from build123d import *

# Parameters (mm, degrees)
EXTRUDE_1_DEPTH      = 13.5
SKETCH_5_R           = 10.1
CUT_EXTRUDE_2_DEPTH  = 1.5
SKETCH_7_R           = 3.5
CUT_EXTRUDE_3_DEPTH  = 37
SKETCH_9_R           = 1.5
CUT_EXTRUDE_4_DEPTH  = 24.5
SKETCH_11_W          = 60.4
SKETCH_11_H          = 24
EXTRUDE_2_DEPTH      = 10
SKETCH_12_R          = 2.7
CUT_EXTRUDE_5_DEPTH  = 8.5
SKETCH_18_R          = 12
CUT_EXTRUDE_9_DEPTH  = 1.5
SKETCH_19_W          = 14.67242397
SKETCH_19_H          = 6
CUT_EXTRUDE_10_DEPTH = 3
SKETCH_20_W          = 76.507524202
SKETCH_20_H          = 37.102074034
CUT_EXTRUDE_11_DEPTH = 3.5


with BuildPart() as part:
    # Sketch 1 → Extrude 1 (new body)
    with BuildSketch(Plane.XY):
        with BuildLine():
            Line((0, 12), (36.185307738, 12))
            Line((36.185307738, 12), (36.185307738, -12))
            Line((36.185307738, -12), (0, -12))
            ThreePointArc((0, -12), (-12, 0), (0, 12))
        make_face()
    extrude(amount=EXTRUDE_1_DEPTH)

    # Sketch 5 → Cut-Extrude 2 (cut)
    with BuildSketch(Plane(origin=(0, 0, 0), x_dir=(-1, 0, 0), z_dir=(0, 0, -1))):
        Circle(SKETCH_5_R)
    extrude(amount=-CUT_EXTRUDE_2_DEPTH, mode=Mode.SUBTRACT)

    # Sketch 7 → Cut-Extrude 3 (cut)
    with BuildSketch(Plane(origin=(0, 0, 1.5), x_dir=(-1, 0, 0), z_dir=(0, 0, -1))):
        Circle(SKETCH_7_R)
    extrude(amount=-CUT_EXTRUDE_3_DEPTH, mode=Mode.SUBTRACT)

    # Sketch 9 → Cut-Extrude 4 (cut)
    with BuildSketch(Plane(origin=(0, 0, 1.5), x_dir=(-1, 0, 0), z_dir=(0, 0, -1))):
        with Locations((-4.949747468, 4.949747468)):
            Circle(SKETCH_9_R)
        with Locations((4.949747468, 4.949747468)):
            Circle(SKETCH_9_R)
        with Locations((4.949747468, -4.949747468)):
            Circle(SKETCH_9_R)
        with Locations((-4.949747468, -4.949747468)):
            Circle(SKETCH_9_R)
    extrude(amount=-CUT_EXTRUDE_4_DEPTH, mode=Mode.SUBTRACT)


with BuildPart() as body_2:
    # Mirror 14: mirrored copy
    add(part.part.mirror(Plane(origin=(0, 0, -16.7), x_dir=(1, 0, 0), z_dir=(0, 0, -1))))


with BuildPart() as part_1:
    add(part.part)

    add(body_2.part)  # Extrude 2 merges body 2
    # Sketch 11 → Extrude 2 (add)
    with BuildSketch(Plane(origin=(36.185307738, 0, 0), x_dir=(0, 0, -1), z_dir=(1, 0, 0))):
        with Locations((16.7, 0)):
            Rectangle(SKETCH_11_W, SKETCH_11_H)
    extrude(amount=-EXTRUDE_2_DEPTH)

    # Sketch 12 → Cut-Extrude 5 (cut)
    with BuildSketch(Plane.XY.offset(13.5)):
        with Locations((4.949747468, 4.949747468)):
            Circle(SKETCH_12_R)
        with Locations((4.949747468, -4.949747468)):
            Circle(SKETCH_12_R)
        with Locations((-4.949747468, -4.949747468)):
            Circle(SKETCH_12_R)
        with Locations((-4.949747468, 4.949747468)):
            Circle(SKETCH_12_R)
    cut_extrude_5 = extrude(amount=-CUT_EXTRUDE_5_DEPTH, mode=Mode.SUBTRACT)

    # Sketch 18 → Cut-Extrude 9 (cut)
    with BuildSketch(Plane(origin=(0, 0, 0), x_dir=(-1, 0, 0), z_dir=(0, 0, -1))):
        Circle(SKETCH_18_R)
    cut_extrude_9 = extrude(amount=-CUT_EXTRUDE_9_DEPTH, mode=Mode.SUBTRACT)

    # Sketch 19 → Cut-Extrude 10 (cut)
    with BuildSketch(Plane(origin=(0, 0, 1.5), x_dir=(-1, 0, 0), z_dir=(0, 0, -1))):
        with Locations((7.336211985, 0)):
            Rectangle(SKETCH_19_W, SKETCH_19_H)
    cut_extrude_10 = extrude(amount=-CUT_EXTRUDE_10_DEPTH, mode=Mode.SUBTRACT)

    # Sketch 20 → Cut-Extrude 11 (cut)
    with BuildSketch(Plane.XY.offset(13.5)):
        with Locations((20.283666709, 0.248055891)):
            Rectangle(SKETCH_20_W, SKETCH_20_H)
    cut_extrude_11 = extrude(amount=-CUT_EXTRUDE_11_DEPTH, mode=Mode.SUBTRACT)

    # Mirror 24: Cut-Extrude 5, Cut-Extrude 9, Cut-Extrude 10 across plane
    add(cut_extrude_5.mirror(Plane(origin=(0, 0, -16.7), x_dir=(1, 0, 0), z_dir=(0, 0, -1))), mode=Mode.SUBTRACT)
    add(cut_extrude_9.mirror(Plane(origin=(0, 0, -16.7), x_dir=(1, 0, 0), z_dir=(0, 0, -1))), mode=Mode.SUBTRACT)
    add(cut_extrude_10.mirror(Plane(origin=(0, 0, -16.7), x_dir=(1, 0, 0), z_dir=(0, 0, -1))), mode=Mode.SUBTRACT)

    # Mirror 26: Cut-Extrude 11 across plane
    add(cut_extrude_11.mirror(Plane(origin=(0, 0, -16.7), x_dir=(1, 0, 0), z_dir=(0, 0, -1))), mode=Mode.SUBTRACT)


solid = part_1.part
Source: CAD feature listing. Evaluate the final solid. Frame: model axes, mm. A direction names the side the tool comes from. Give positions to 0.01 mm unless a question says otherwise; leave off trailing zeros. Write each loop counter-clockwise with the first axis right and the second up, starting at its lowest first coordinate (ties: lowest second). Pieces come first, ordered by that corner, then holes. Notation, with made-up numbers: (62, 40) - (95, 40) arc R6 cw to (95, 48) - close; hole circle Ø7 at (80, -35). An arc over 180 degrees is marked (long way). Write item = value, one per line. Start each with the question number.
Q1. Cut plane B-B, the plane x = 13.5. Return loops of the section in (y, z).
Q2. Cut plane C-C, the plane z = -37. Return loops of the section in (x, y).
Q3. Reachability of faces 4 (the cylindrical face through (6.14, 4.04, -36.63)), 5 (the flat face through (-8, 0, -37.9)), 6 (the cylindrical face through (4.364, -7.586, 7.535)), 7 (the flat face through (5, -7, -38.4)), 8 (the flat face through (19, 0, 0)) from +Z, -Z, +X, -X, +Y, -Y: full face, straight path, thin tool, end or side. Return the list, or none.
Q4. Pin query (flat end, axial travel): pin 1 Ø2.5 at (x, y) = (-5.5, -6) entering from +Z; pin 2 Ø2.5 at (x, z) = (-5.5, -37) entering from +Y; pin 3 Ø3.5 at (x, y) = (-4.95, 4.95) entering from -Z. Return the tip coordinate at first contact, or that it passes through.
Q5. Cut plane A-A, the plane y = 0. Return loops of the section in (x, z).
Q6. Material intervals for probe 1 along Z at (x, y) = (7, -0.5); probe 2 along Z at (x, y) = (24, 9.5); probe 3 along X at (y, z) = (-2.75, 7.5), sorted ascending.
Q7. Draft query along Y for faces 1 (the flat face through (-5, 3, -38.4)), 2 (the flat face through (17, 0, -43.4)), 3 (the flat face through (26.4, -12, -17.1)). Return one class per face: +Y half, -Y half, draft (parallel to the pull), parting line (faces both ways), or undercut.
Computed values:
q1.outline = (-12, -43.4) - (12, -43.4) - (12, -33.4) - (-12, -33.4) - close; (-12, 0) - (12, 0) - (12, 10) - (-12, 10) - close
q2.outline = (-11.62, -3) arc R12 ccw to (0, -12) - (36.19, -12) - (36.19, 12) - (0, 12) arc R12 ccw to (-11.62, 3) - (-1.8, 3) arc R3.5 cw (long way) to (-1.8, -3) - close; hole circle Ø3 at (-4.95, -4.95); hole circle Ø3 at (-4.95, 4.95); hole circle Ø3 at (4.95, -4.95); hole circle Ø3 at (4.95, 4.95)
q3.face_4 = +Z, -Z
q3.face_5 = -X
q3.face_6 = +Z
q3.face_7 = -Z
q3.face_8 = -X, +Y, -Y
q4.pin_1 = 5
q4.pin_2 = 11.22
q4.pin_3 = -38.4
q5.outline = (-12, -43.4) - (-3.5, -43.4) - (-3.5, -37.9) - (-12, -37.9) - close; (-12, 4.5) - (-3.5, 4.5) - (-3.5, 10) - (-12, 10) - close; (3.5, -43.4) - (36.19, -43.4) - (36.19, 10) - (3.5, 10) - (3.5, 1.5) - (12, 1.5) - (12, 0) - (26.19, 0) - (26.19, -33.4) - (12, -33.4) - (12, -34.9) - (3.5, -34.9) - close
q6.probe_1 = -43.4 to -34.9, 1.5 to 10
q6.probe_2 = -43.4 to -33.4, 0 to 10
q6.probe_3 = -11.68 to -6.52, -3.38 to -2.17, 2.17 to 3.38, 6.52 to 36.19
q7.face_1 = undercut
q7.face_2 = draft
q7.face_3 = -Y half
